Here's how the part is built. I have some questions about the finished solid (model axes, mm). A direction names the side the tool comes from. Coordinates: 2 decimals unless noted, no trailing zeros. Write each loop counter-clockwise with the first axis right and the second up, starting at its lowest first coordinate (ties: lowest second). Pieces come first, ordered by that corner, then holes.
(1) Please list where these lines run through material, in increasing order: probe 1 along Z at (x, y) = (21, -6); probe 2 along X at (y, z) = (-2.25, 24.5); probe 3 along Z at (x, y) = (16, -5.5).
(2) Imagine slicing it at A-A, the plane z = -55. List the corners of the cut face in (x, y) for me.
(3) Imagine slicing it at C-C, the plane z = 55. List the corners of the cut face in (x, y) for me, plus the area to 3 significant figures.
(4) Which directions (+Z, -Z, +X, -X, +Y, -Y) give clear straight access to the entire face, cutting with the end or side of a thin tool? Please do faces 4 (the flat face through (-20, -6, 36)), 5 (the cylindrical face through (0.42, -3.615, -54.249)).
(5) For pin 1 Ø4.5 at (y, z) = (-6, 55) entering from +X; pin 2 Ø5 at (x, z) = (-17.5, -27.5) entering from +Y, each with a flat end and sliding along its axis, tell me the tip position at first contact or that it passes through.
(6) Thinking about a two-plate mould opening in Z: for faces 1 (the cylindrical face through (15.21, -3.615, 55.751)), 2 (the flat face through (30, -6, -1)), 3 (the flat face through (0, -6, -60)), which applies, released by +Z, released by -Z, zero draft, split by the parting line, or undercut?
(7) Imagine slicing it at B-B, the plane y = -6. List the corners of the cut face in (x, z) for me.
(8) Imagine slicing it at D-D, the plane x = -9.5. List the corners of the cut face in (y, z) for me.
```python
from build123d import *

# Parameters (mm, degrees)
F0_W     = 60
F0_H     = 120
F2_DEPTH = 12
F1_W     = 20
F1_H     = 48
F3_DEPTH = 12
F4_R     = 2.5
F5_DEPTH = 60.001
F6_R     = 2.5
F7_DEPTH = 152.4


with BuildPart() as f2:
    # F0 (on Front) → F2 (new body)
    with BuildSketch(Plane.XZ):
        Rectangle(F0_W, F0_H)
    extrude(amount=F2_DEPTH)

    # F1 (on face) → F3 (cut, through all)
    with BuildSketch(Plane.XZ):
        with Locations((-10, 36)):
            Rectangle(F1_W, F1_H)
    extrude(amount=F3_DEPTH, mode=Mode.SUBTRACT)

    # F4 (on face) → F5 (cut, through all)
    with BuildSketch(Plane.YZ.offset(30)):
        with Locations((-6, 55)):
            Circle(F4_R)
    extrude(amount=-F5_DEPTH, mode=Mode.SUBTRACT)

    # F6 (on face) → F7 (cut)
    with BuildSketch(Plane.YZ.offset(30)):
        with Locations((-6, -55)):
            Circle(F6_R)
    extrude(amount=-F7_DEPTH, mode=Mode.SUBTRACT)


solid = f2.part
```
Recorded:
1. probe 1: z = -60 to -57.5, -52.5 to 52.5, 57.5 to 60
1. probe 2: x = -30 to -20, 0 to 30
1. probe 3: z = -60 to -57.45, -52.55 to 52.55, 57.45 to 60
2. outline: (-30, -12) - (30, -12) - (30, -8.5) - (-30, -8.5) - close; (-30, -3.5) - (30, -3.5) - (30, 0) - (-30, 0) - close
3. outline: (-30, -12) - (-20, -12) - (-20, -8.5) - (-30, -8.5) - close; (-30, -3.5) - (-20, -3.5) - (-20, 0) - (-30, 0) - close; (0, -12) - (30, -12) - (30, -8.5) - (0, -8.5) - close; (0, -3.5) - (30, -3.5) - (30, 0) - (0, 0) - close
3. area: 280 mm2
4. face 4: +Z, +Y, -Y
4. face 5: +X, -X
5. pin 1: passes through
5. pin 2: stops at y = 0
6. face 1: undercut
6. face 2: zero draft
6. face 3: released by -Z
7. outline: (-30, -60) - (30, -60) - (30, -57.5) - (-30, -57.5) - close; (-30, -52.5) - (30, -52.5) - (30, 52.5) - (0, 52.5) - (0, 12) - (-20, 12) - (-20, 52.5) - (-30, 52.5) - close; (-30, 57.5) - (-20, 57.5) - (-20, 60) - (-30, 60) - close; (0, 57.5) - (30, 57.5) - (30, 60) - (0, 60) - close
8. outline: (-12, -60) - (0, -60) - (0, 12) - (-12, 12) - close; hole circle Ø5 at (-6, -55)
